Verification items for the finished model (mm, model axes). Face numbers are marked on the shaded views. Coordinates: 2 decimals unless noted, no trailing zeros. Write each loop counter-clockwise with the first axis right and the second up, starting at its lowest first coordinate (ties: lowest second). Pieces come first, ordered by that corner, then holes. Notation, with made-up numbers: (-28.75, 35.5) -> (-15.75, 35.5) arc R21 ccw to (-15.75, 47.5) -> close; hole circle Ø7 at (7, 87.25). An arc over 180 degrees is marked (long way). Answer in a Markdown table with one row per item.
```python
from build123d import *

# Parameters (mm, degrees)
F1_DEPTH = 35
F2_R     = 6.5
F4_DEPTH = 3.5
F2_R_2   = 4.65
F5_DEPTH = 4
F3_R     = 6.5
F6_DEPTH = 3
F3_R_2   = 5
F7_DEPTH = 5


with BuildPart() as f1:
    # F0 (on Top) → F1 (new body)
    with BuildSketch(Plane.XY):
        with BuildLine():
            Line((18.748637, 81.127049), (18.748637, 91.127049))
            Line((18.748637, 91.127049), (-6.251363, 91.127049))
            ThreePointArc((-6.251363, 91.127049), (-9.786897, 89.662583), (-11.251363, 86.127049))
            Line((-11.251363, 86.127049), (-11.251363, -93.872951))
            ThreePointArc((-11.251363, -93.872951), (-9.786897, -97.408485), (-6.251363, -98.872951))
            Line((-6.251363, -98.872951), (18.748637, -98.872951))
            Line((18.748637, -98.872951), (18.748637, -88.872951))
            ThreePointArc((18.748637, -88.872951), (17.284171, -85.337417), (13.748637, -83.872951))
            Line((13.748637, -83.872951), (8.748637, -83.872951))
            ThreePointArc((8.748637, -83.872951), (5.213103, -82.408485), (3.748637, -78.872951))
            Line((3.748637, -78.872951), (3.748637, 71.127049))
            ThreePointArc((3.748637, 71.127049), (5.213103, 74.662583), (8.748637, 76.127049))
            Line((8.748637, 76.127049), (13.748637, 76.127049))
            ThreePointArc((13.748637, 76.127049), (17.284171, 77.591515), (18.748637, 81.127049))
        make_face()
    extrude(amount=F1_DEPTH)

    # F2 (on face) → F4 (cut)
    with BuildSketch(Plane.XY.offset(35)):
        with Locations((-1.251363, 81.127049)):
            Circle(F2_R)
        with Locations((-1.251363, -88.872951)):
            Circle(F2_R)
    extrude(amount=-F4_DEPTH, mode=Mode.SUBTRACT)

    # F2 (on face) → F5 (join)
    with BuildSketch(Plane.XY.offset(35)):
        with Locations((-3.751363, 61.127049)):
            Circle(F2_R_2)
        with Locations((-3.751363, -68.872951)):
            Circle(F2_R_2)
    extrude(amount=F5_DEPTH)

    # F3 (on face) → F6 (cut)
    with BuildSketch(Plane(origin=(0, 0, 0), x_dir=(1, 0, 0), z_dir=(0, 0, -1))):
        with Locations((-1.251363, -81.127049)):
            Circle(F3_R)
        with Locations((-1.251363, 88.872951)):
            Circle(F3_R)
    extrude(amount=-F6_DEPTH, mode=Mode.SUBTRACT)

    # F3 (on face) → F7 (cut)
    with BuildSketch(Plane(origin=(0, 0, 0), x_dir=(1, 0, 0), z_dir=(0, 0, -1))):
        with Locations((-3.751363, -61.127049)):
            Circle(F3_R_2)
        with Locations((-3.751363, 68.872951)):
            Circle(F3_R_2)
    extrude(amount=-F7_DEPTH, mode=Mode.SUBTRACT)


solid = f1.part
```
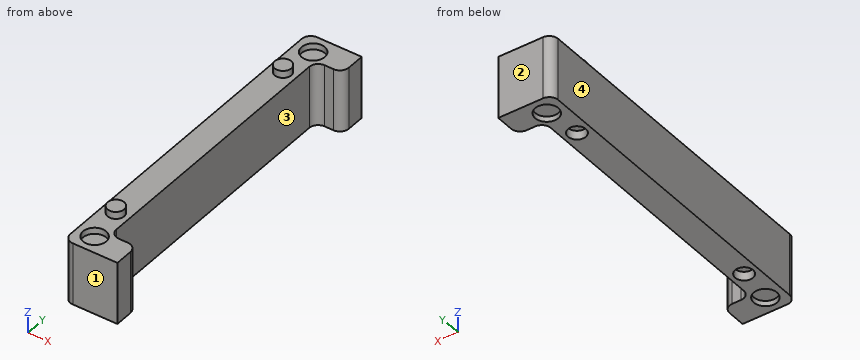
1. Section check A-A, the plane x = 11. Record the boundary of the cut face in (y, z).
Geometry says:
| item | result |
|---|---|
| outline | (-98.87, 0) -> (-83.87, 0) -> (-83.87, 35) -> (-98.87, 35) -> close; (76.13, 0) -> (91.13, 0) -> (91.13, 35) -> (76.13, 35) -> close |
2. Mould release check, pull along Y, two halves, no side actions. Record for the marked faces 1, 2, 3 and 4: released by +Y, released by -Y, zero draft, split by the parting line, or undercut.
Geometry says:
| item | result |
|---|---|
| face 1 | released by -Y |
| face 2 | released by +Y |
| face 3 | undercut |
| face 4 | zero draft |
3. Depth check by flat-ended pin: P1, Ø14.5, axis at x = -0.5, y = -86, coming from the +Z side; P2, Ø17, axis at x = -1.25, y = -88.87, coming from the -Z side; P3, Ø6, axis at x = -3.75, y = -68.87, coming from the -Z side; P4, Ø1.5, axis at y = -65, z = 6, coming from the +X side. Enter the tip coordinate at first touch or a pass-through.
Geometry says:
| item | result |
|---|---|
| P1 | z = 35 |
| P2 | z = 0 |
| P3 | z = 5 |
| P4 | x = 3.75 |
4. Section check B-B, the plane z = 14.5. Record the boundary of the cut face in (x, y).
Geometry says:
| item | result |
|---|---|
| outline | (-11.25, -93.87) arc R5 ccw to (-6.25, -98.87) -> (18.75, -98.87) -> (18.75, -88.87) arc R5 ccw to (13.75, -83.87) -> (8.75, -83.87) arc R5 cw to (3.75, -78.87) -> (3.75, 71.13) arc R5 cw to (8.75, 76.13) -> (13.75, 76.13) arc R5 ccw to (18.75, 81.13) -> (18.75, 91.13) -> (-6.25, 91.13) arc R5 ccw to (-11.25, 86.13) -> close |
5. Section check D-D, the plane y = 21. Record the boundary of the cut face in (x, z).
Geometry says:
| item | result |
|---|---|
| outline | (-11.25, 0) -> (3.75, 0) -> (3.75, 35) -> (-11.25, 35) -> close |
6. Thickness scan on line 1 (Y direction, x = 11.5, z = 18.5); line 2 (Z direction, x = -9, y = 80); line 3 (X direction, y = 66, z = 24). Record the ranges inside material, lowest first. Write a range as from..to.
Geometry says:
| item | result |
|---|---|
| line 1 | -98.87..-83.87, 76.13..91.13 |
| line 2 | 0..35 |
| line 3 | -11.25..3.75 |
7. Section check C-C, the plane y = -87. Record the boundary of the cut face in (x, z), plus the area to 3 significant figures.
Geometry says:
| item | result |
|---|---|
| outline | (-11.25, 0) -> (-7.48, 0) -> (-7.48, 3) -> (4.97, 3) -> (4.97, 0) -> (18.38, 0) -> (18.38, 35) -> (4.97, 35) -> (4.97, 31.5) -> (-7.48, 31.5) -> (-7.48, 35) -> (-11.25, 35) -> close |
| area | 956 mm^2 |
